from build123d import *

# Parameters (mm, degrees)
F0_W     = 69.85
F0_H     = 69.85
F0_R     = 1.6383
F1_DEPTH = 1.5748
F2_W     = 8.2296
F2_H     = 31.75
F3_DEPTH = 27.94
F4_W     = 10.16
F4_H     = 6.7056
F5_DEPTH = 13.97


with BuildPart() as f1:
    # F0 (on Top) → F1 (new body)
    with BuildSketch(Plane.XY):
        Rectangle(F0_W, F0_H)
        with Locations((-31.115, -31.115)):
            Circle(F0_R, mode=Mode.SUBTRACT)
        with Locations((31.115, -31.115)):
            Circle(F0_R, mode=Mode.SUBTRACT)
        with Locations((-31.115, 31.115)):
            Circle(F0_R, mode=Mode.SUBTRACT)
        with Locations((31.115, 31.115)):
            Circle(F0_R, mode=Mode.SUBTRACT)
    extrude(amount=F1_DEPTH)

    # F2 (on face) → F3 (join)
    with BuildSketch(Plane.XY.offset(1.5748)):
        with Locations((-28.575, 10.16)):
            Rectangle(F2_W, F2_H)
    extrude(amount=F3_DEPTH)

    # F4 (on face) → F5 (join)
    with BuildSketch(Plane.XY.offset(1.5748)):
        with Locations((-21.717, -16.9418)):
            Rectangle(F4_W, F4_H)
        with Locations((-5.207, -16.9418)):
            Rectangle(F4_W, F4_H)
    extrude(amount=F5_DEPTH)


solid = f1.part
Model file for the job. Use its own axes, mm. A direction names the side the tool comes from. Coordinates: 2 decimals unless noted, no trailing zeros. Loops run counter-clockwise (first coordinate to the right, second up) from the corner with the lowest first, then second, coordinate; pieces in that order, holes last. Notation, with made-up numbers: (9.5, -20.75) -> (60.5, -20.75) arc R29 ccw to (60.5, 14.25) -> close; hole circle Ø9 at (1.5, 64.25). An arc over 180 degrees is marked (long way). Use one line per item in the form item = value. Start each with the question number.
(1) Cut at C-C on y = -7.5. Give the cut face in (x, z) (3 decimals).
(2) Flat gauge pins, fed straight in: pin 1 (5.5 mm diameter, centred on x = -21, y = -17.5, fed in from +Z); pin 2 (1.5 mm diameter, centred on y = 7.5, z = 15, fed in from +X); pin 3 (4 mm diameter, centred on x = 31.115, y = 31.115, fed in from +Z). Where does each tip first touch, or does it go through?
(3) Cut at B-B on x = -6. Give the cut face in (y, z) (3 decimals), and give its area (3 significant figures).
(4) Cut at D-D on z = 22.5. Give the cut face in (x, y) (3 decimals).
(5) Pull direction Y, two halves, no side cores. Call faces 1 (the flat face through (-32.69, 10, 15)), 2 (the cylindrical face through (29.815, 30.118, 0.776)), 3 (the flat face through (-22, -20.295, 8)): pulls with the +Y half, pulls with the -Y half, needs draft (parallel to the pull), parting line crosses it, or undercut.
(6) Tool access for faces 4 (the flat face through (-0.127, -17, 8)), 5 (the flat face through (-5, -20.295, 8)), 6 (the flat face through (-22, -13.589, 8)), 7 (the flat face through (-5, -13.589, 8)), 8 (the flat face through (-24.46, 10, 15)): list every direction of +Z, -Z, +X, -X, +Y, -Y with a clear straight run to the whole face (end or side of a thin tool).
(7) Cut at A-A on z = 13.75. Give the cut face in (x, y) (3 decimals), and give its area (3 significant figures).
(8) Probe probe 1 along X at (y, z) = (-17, 11.5); probe 2 along Z at (x, y) = (14.5, -17); probe 3 along X at (y, z) = (12, 9). List the from-to ranges inside material, lowest first. Write a range as from..to.
Values:
q1.outline = (-34.925, 0) -> (34.925, 0) -> (34.925, 1.575) -> (-34.925, 1.575) -> close
q2.pin_1 = 15.54
q2.pin_2 = -24.46
q2.pin_3 = 1.57
q3.outline = (-34.925, 0) -> (34.925, 0) -> (34.925, 1.575) -> (-13.589, 1.575) -> (-13.589, 15.545) -> (-20.295, 15.545) -> (-20.295, 1.575) -> (-34.925, 1.575) -> close
q3.area = 204 mm2
q4.outline = (-32.69, -5.715) -> (-24.46, -5.715) -> (-24.46, 26.035) -> (-32.69, 26.035) -> close
q5.face_1 = needs draft
q5.face_2 = undercut
q5.face_3 = pulls with the -Y half
q6.face_4 = +Z, +X, +Y, -Y
q6.face_5 = +Z, +X, -X, -Y
q6.face_6 = +Z, +X, -X
q6.face_7 = +Z, +X, -X, +Y
q6.face_8 = +Z, +X, +Y
q7.outline = (-32.69, -5.715) -> (-24.46, -5.715) -> (-24.46, 26.035) -> (-32.69, 26.035) -> close; (-26.797, -20.295) -> (-16.637, -20.295) -> (-16.637, -13.589) -> (-26.797, -13.589) -> close; (-10.287, -20.295) -> (-0.127, -20.295) -> (-0.127, -13.589) -> (-10.287, -13.589) -> close
q7.area = 398 mm2
q8.probe_1 = -26.8..-16.64, -10.29..-0.13
q8.probe_2 = 0..1.57
q8.probe_3 = -32.69..-24.46
